Part print with two shaded views. Sizes in mm from the minimum x, y, z corner. A direction names the side the tool comes from. Round coordinates to 2 decimals unless told otherwise and drop trailing zeros. Order: outer loops, then holes, each group sorted by start corner. A loop starts at its lowest first (then second) coordinate and runs counter-clockwise, first axis right, second up. Notation, with made-up numbers: (-11.5, 89) - (30.5, 89) arc R22 ccw to (30.5, 101) - close; hole circle Ø10 at (-23.75, -5). An arc over 180 degrees is marked (long way). Use one line per item in the form item = value.
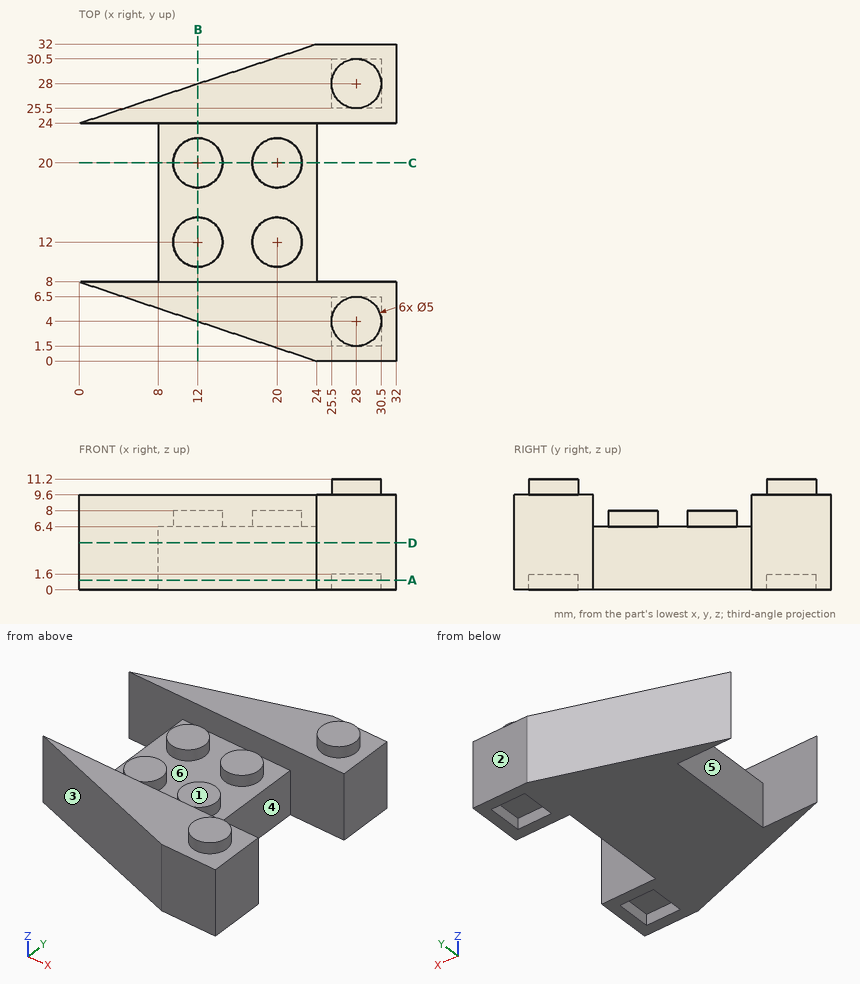
(1) Slice it at D-D on z = 4.75. Give the cut face in (x, y), then the cut area to 3 significant figures.
Report:
outline = (0, 8) - (24, 0) - (32, 0) - (32, 8) - (24, 8) - (24, 24) - (32, 24) - (32, 32) - (24, 32) - (0, 24) - (8, 24) - (8, 8) - close
area = 576 mm2
(2) Slice it at A-A on z = 1. Give the cut face in (x, y), then the cut area to 3 significant figures.
Report:
outline = (0, 8) - (24, 0) - (32, 0) - (32, 8) - (24, 8) - (24, 24) - (32, 24) - (32, 32) - (24, 32) - (0, 24) - (8, 24) - (8, 8) - close; hole (25.5, 1.5) - (30.5, 1.5) - (30.5, 6.5) - (25.5, 6.5) - close; hole (25.5, 25.5) - (30.5, 25.5) - (30.5, 30.5) - (25.5, 30.5) - close
area = 526 mm2
(3) Probe probe 1 along Y at (x, z) = (4.5, 8); probe 2 along X at (y, z) = (17.5, 2.25); probe 3 along Y at (x, z) = (15.5, 8.25). List the from-to ranges inside material, lowest first. Write a range as [from, to].
Report:
probe_1 = [6.5, 8], [24, 25.5]
probe_2 = [8, 24]
probe_3 = [2.83, 8], [24, 29.17]
(4) Pull direction Y, two halves, no side cores. Call the marked faces 1, 2 and 3: released by +Y, released by -Y, zero draft, split by the parting line, or undercut.
Report:
face_1 = undercut
face_2 = released by +Y
face_3 = released by -Y
(5) Slice it at C-C on y = 20. Give the cut face in (x, z).
Report:
outline = (8, 0) - (24, 0) - (24, 6.4) - (22.5, 6.4) - (22.5, 8) - (17.5, 8) - (17.5, 6.4) - (14.5, 6.4) - (14.5, 8) - (9.5, 8) - (9.5, 6.4) - (8, 6.4) - close
(6) Pin check, flat tips, straight feed: pin 1 (4 mm diameter, centred on x = 22, y = 9.5, fed in from +Z); pin 2 (5 mm diameter, centred on x = 10, z = 6, fed in from -Y); pin 3 (3 mm diameter, centred on x = 26, y = 15.5, fed in from -Z) (3 decimals); pin 4 (1.5 mm diameter, centred on x = 13, y = 20, fed in from +Z). Stop position of each tip, or through.
Report:
pin_1 = 9.6
pin_2 = 3.83
pin_3 = through
pin_4 = 8
(7) Tool access for the marked faces 4, 5 and 6: list every direction of +Z, -Z, +X, -X, +Y, -Y with a clear straight run to the whole face (end or side of a thin tool).
Report:
face_4 = +Z, -Z, +X
face_5 = +Z, -Z, -X
face_6 = +Z
(8) Slice it at B-B on x = 12. Give the cut face in (y, z), then the cut area to 3 significant figures.
Report:
outline = (4, 0) - (28, 0) - (28, 9.6) - (24, 9.6) - (24, 6.4) - (22.5, 6.4) - (22.5, 8) - (17.5, 8) - (17.5, 6.4) - (14.5, 6.4) - (14.5, 8) - (9.5, 8) - (9.5, 6.4) - (8, 6.4) - (8, 9.6) - (4, 9.6) - close
area = 195 mm2
